from build123d import *

# Parameters (mm, degrees)
SKETCH1_R           = 30.5
SKETCH1_R_2         = 22.025
BOSS_EXTRUDE1_DEPTH = 3.5
LAPVSROTOR_START    = 3.5
SKETCH1_8_R         = 29.25
SKETCH1_8_R_2       = 22.025
LAPVSROTOR_DEPTH    = 10
CUT_EXTRUDE1_START  = 13.5
SKETCH1_9_R         = 1.55
CUT_EXTRUDE1_DEPTH  = 10
SKETCH2_R           = 22.05
SKETCH2_R_2         = 21
BOSS_EXTRUDE3_DEPTH = 1
SKETCH3_R           = 1.55
CUT_EXTRUDE2_DEPTH  = 46.196791922
CUT_EXTRUDE3_START  = 7.5
SKETCH4_R           = 28.075
SKETCH4_R_2         = 21
CUT_EXTRUDE3_DEPTH  = 6
SKETCH5_R           = 3
CUT_EXTRUDE4_DEPTH  = 2.5
CHAMFER1_SIZE       = 0.5
CIRPATTERN1_COUNT   = 7


with BuildPart() as part:
    # Sketch1 → Boss-Extrude1 (new body)
    with BuildSketch(Plane.XY):
        Circle(SKETCH1_R)
        Circle(SKETCH1_R_2, mode=Mode.SUBTRACT)
    extrude(amount=BOSS_EXTRUDE1_DEPTH)

    # Sketch1<8> → lapvsrotor (add)
    with BuildSketch(Plane.XY.offset(LAPVSROTOR_START)):
        Circle(SKETCH1_8_R)
        Circle(SKETCH1_8_R_2, mode=Mode.SUBTRACT)
    extrude(amount=LAPVSROTOR_DEPTH)

    # Sketch1<9> → Cut-Extrude1 (cut)
    with BuildSketch(Plane.XY.offset(CUT_EXTRUDE1_START)):
        with Locations((0, 25)):
            Circle(SKETCH1_9_R)
        with Locations((10.847093478, 22.524221698)):
            Circle(SKETCH1_9_R)
        with Locations((19.545787062, 15.587245046)):
            Circle(SKETCH1_9_R)
        with Locations((24.373197805, 5.563023349)):
            Circle(SKETCH1_9_R)
        with Locations((24.373197805, -5.563023349)):
            Circle(SKETCH1_9_R)
        with Locations((19.545787062, -15.587245046)):
            Circle(SKETCH1_9_R)
        with Locations((10.847093478, -22.524221698)):
            Circle(SKETCH1_9_R)
        with Locations((0, -25)):
            Circle(SKETCH1_9_R)
        with Locations((-10.847093478, -22.524221698)):
            Circle(SKETCH1_9_R)
        with Locations((-19.545787062, -15.587245046)):
            Circle(SKETCH1_9_R)
        with Locations((-24.373197805, -5.563023349)):
            Circle(SKETCH1_9_R)
        with Locations((-24.373197805, 5.563023349)):
            Circle(SKETCH1_9_R)
        with Locations((-19.545787062, 15.587245046)):
            Circle(SKETCH1_9_R)
        with Locations((-10.847093478, 22.524221698)):
            Circle(SKETCH1_9_R)
    extrude(amount=-CUT_EXTRUDE1_DEPTH, mode=Mode.SUBTRACT)

    # Sketch2 → Boss-Extrude3 (add)
    with BuildSketch(Plane.XY):
        Circle(SKETCH2_R)
        Circle(SKETCH2_R_2, mode=Mode.SUBTRACT)
    extrude(amount=BOSS_EXTRUDE3_DEPTH)

    # Sketch3 → Cut-Extrude2 (cut, through all)
    with BuildSketch(Plane.XY):
        with Locations((5.89680475, 25.835589673)):
            Circle(SKETCH3_R)
        with Locations((23.875674999, 11.497919087)):
            Circle(SKETCH3_R)
        with Locations((23.875674999, -11.497919087)):
            Circle(SKETCH3_R)
        with Locations((5.89680475, -25.835589673)):
            Circle(SKETCH3_R)
        with Locations((-16.522479749, -20.718534285)):
            Circle(SKETCH3_R)
        with Locations((-26.5, 0)):
            Circle(SKETCH3_R)
        with Locations((-16.522479749, 20.718534285)):
            Circle(SKETCH3_R)
    extrude(amount=CUT_EXTRUDE2_DEPTH, mode=Mode.SUBTRACT)

    # Sketch4 → Cut-Extrude3 (cut)
    with BuildSketch(Plane.XY.offset(CUT_EXTRUDE3_START)):
        Circle(SKETCH4_R)
        Circle(SKETCH4_R_2, mode=Mode.SUBTRACT)
    extrude(amount=CUT_EXTRUDE3_DEPTH, mode=Mode.SUBTRACT)

    # Sketch5 → Cut-Extrude4 (cut)
    with BuildSketch(Plane.XY):
        with Locations((5.89680475, 25.835589673)):
            Circle(SKETCH5_R)
    cut_extrude4 = extrude(amount=CUT_EXTRUDE4_DEPTH, mode=Mode.SUBTRACT)

    # Chamfer1
    chamfer1_edges = [part.edges().sort_by_distance(p)[0] for p in [
        (-22.025, 0, 7.5),
        (-30.5, 0, 0),
        (-29.25, 0, 13.5),
    ]]
    chamfer(chamfer1_edges, length=CHAMFER1_SIZE)

    # CirPattern1: Cut-Extrude4 ×7 about axis
    cirpattern1_axis = Axis((0, 0, 0), (0, 0, 1))
    for i in range(1, CIRPATTERN1_COUNT):
        add(cut_extrude4.rotate(cirpattern1_axis, i * 360 / CIRPATTERN1_COUNT), mode=Mode.SUBTRACT)


solid = part.part
The listing builds one solid part. Answer for the finished solid, in the listing's coordinates (mm). A direction names the side the tool comes from. Give positions to 0.01 mm unless a question says otherwise; leave off trailing zeros. Write each question's results on one line, items separated by ' | '.
1. Which of the six approach directions +Z, -Z, +X, -X, +Y, -Y give full straight-line access (tool end or side, diameter ignored) to faces 1 (the face through (21.008, 6.616, 3.958)), 2 (the face through (-14.7, 20.9, 2.5))?
Resolved:
face 1: +Z | face 2: -Z
2. Consider probe 1 along Y at (x, z) = (25, 6.75); probe 2 along Y at (x, z) = (-17, 8); probe 3 along X at (y, z) = (20, 6.25) (3 decimals). Determine where each line is inside the solid, lowest interval first. Write a range as from..to.
Resolved:
probe 1: y = -15.18..-12.56, -10.43..-6.98, -4.15..4.15, 6.98..10.43, 12.56..15.18 | probe 2: y = -23.8..-22.34, 22.34..23.8 | probe 3: x = -21.344..-17.896, -15.149..-9.225, 9.225..21.344
3. Flat-ended cylindrical pins translate along their axes: P1, Ø1.9, axis at x = 10.85, y = 22.52, coming from the +Z side; P2, Ø3, axis at x = 24.5, y = 12, coming from the -Z side; P3, Ø6, axis at x = -20, z = 7, coming from the -Y side. Find the tip coordinate at first contact, or state that the pin passes through.
Resolved:
P1: stops at z = 3.5 | P2: stops at z = 2.5 | P3: stops at y = -23.8
4. For a pull along Y with two mould halves and no side action, classify faces 3 (the face through (-24.204, -18.559, 1.979)), 4 (the face through (25, -16, 3.5)), 5 (the face through (23.7, 9.7, 2.5)) as +Y half, -Y half, draft (parallel to the pull), parting line (faces both ways), or undercut.
Resolved:
face 3: parting line | face 4: draft | face 5: undercut
5. Find section B-B, the plane y = 0. Count the separate pieces of the cut face and the enclosed holes in it, then the cut area to 3 significant figures.
Resolved:
separate pieces: 3 | enclosed holes: 0 | area: 102 mm^2
